Can you work these out from the model? Positions are in its coordinate system, mm. Face numbers are marked on the shaded views. A direction names the side the tool comes from. Coordinates: 2 decimals unless noted, no trailing zeros. Loops run counter-clockwise (first coordinate to the right, second up) from the corner with the lowest first, then second, coordinate; pieces in that order, holes last.
Autodesk Inventor part; units mm, degrees
ref_plane "XZ Plane" through (0, 0, 0) normal (0, 1, 0) x (-1, 0, 0)
ref_plane "XY Plane" through (0, 0, 0) normal (0, 0, 1) x (1, 0, 0)
ref_plane "Work Plane1" through (30.48, 0, 0) normal (1, 0, 0) x (0, 1, 0)
sketch "Sketch1" plane through (30.48, 0, 0) normal (1, 0, 0) x (0, 1, 0)
  line L0 (-20.1241, -2.3129) -> (-38.2674, 53.7867)
  line L1 (-38.2674, 53.7867) -> (-31.5623, 117.8336)
  line L2 (-31.5623, 117.8336) -> (-5.4691, 117.8336)
  line L3 (-5.4691, 117.8336) -> (117.3937, -58.5065)
  line L4 (117.3937, -58.5065) -> (101.0815, -66.2557)
  line L5 (19.6952, -2.3129) -> (-20.1241, -2.3129)
  line L6 (101.0815, -66.2557) -> (43.3079, -39.3441)
  line L7 (43.3079, -39.3441) -> (19.6952, -2.3129)
  line L8 (-37.8354, 57.9131) -> (-33.5614, 98.738)
  point P0 (0, 0)
  point P1 (-12.6907, 108.8336)
  point P2 (0, 0)
  dimension "d1" = 9
  dimension "d2" = 39.8192
  dimension "d3" = 107.922
  dimension "d5" = 56.0996
  dimension "d6" = 84.023
  dimension "d7" = 64.0469
  dimension "d8" = 26.0932
  dimension "d9" = 55.134
  dimension "d10" = 176.3401
  dimension "d11" = 37.0312
  dimension "d12" = 26.9116
  dimension "d13" = 18.8716
  dimension "d14" = 111.1466
extrude "Extrusion1" add sketch "Sketch1" along normal blind 3.175
ref_plane "Work Plane2" through (-30.48, 0, 0) normal (1, 0, 0) x (0, 1, 0)
sketch "Sketch2" plane through (-30.48, 0, 0) normal (1, 0, 0) x (0, 1, 0)
  line L0 (-20.1241, -2.3129) -> (19.6952, -2.3129)
  line L1 (19.6952, -2.3129) -> (43.3079, -39.3441)
  line L2 (43.3079, -39.3441) -> (101.0815, -66.2557)
  line L3 (101.0815, -66.2557) -> (117.3937, -58.5065)
  line L4 (117.3937, -58.5065) -> (-5.4691, 117.8336)
  line L5 (-5.4691, 117.8336) -> (-31.5623, 117.8336)
  line L6 (-31.5623, 117.8336) -> (-38.2674, 53.7867)
  line L7 (-38.2674, 53.7867) -> (-20.1241, -2.3129)
  point P0 (0, 0)
extrude "Extrusion2" add sketch "Sketch2" against normal blind 3.175
sketch "Sketch3" plane through (0, 0, 0) normal (0, 0, 1) x (1, 0, 0)
  line L0 (-30.48, -12.7) -> (30.48, -12.7)
  line L1 (30.48, -12.7) -> (30.48, 32.385)
  line L2 (30.48, 32.385) -> (-30.48, 32.385)
  line L3 (-30.48, 32.385) -> (-30.48, -12.7)
  line L4 (-30.48, 117.3937) -> (-30.48, -5.4691)
  line L5 (30.48, 117.3937) -> (30.48, -5.4691)
  point P0 (0, 0)
  dimension "d20" = 12.7
  dimension "d21" = 32.385
extrude "Extrusion3" add sketch "Sketch3" along normal blind 3.175
properties part number "ShoulderBoundingBox"
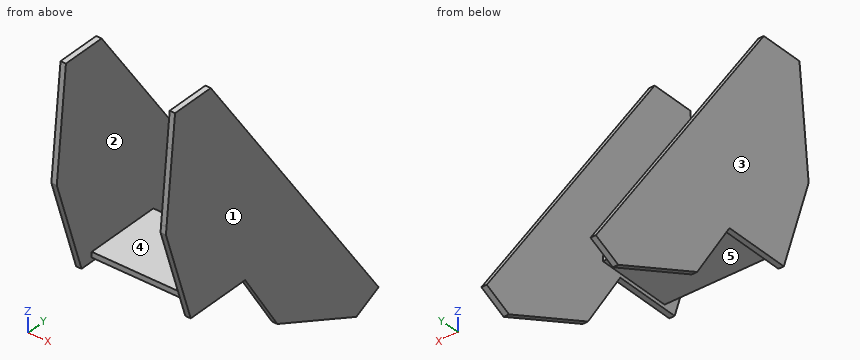
Item 1: I'm going to push flat-ended pins straight in: P1, Ø1, axis at x = -32, y = 7.5, coming from the -Z side; P2, Ø8, axis at x = 17.5, y = 4.5, coming from the +Z side (3 decimals); P3, Ø3.5, axis at x = 9, z = 1, coming from the +Y side (3 decimals). Where does each tip first touch, or does it pass through?
Results are:
P1: stops at z = -2.31
P2: stops at z = 3.175
P3: stops at y = 32.385
Item 2: We'd pull the mould along X, two halves only. Please class the marked faces 1, 2 and 3: +X half, -X half, draft (parallel to the pull), parting line (faces both ways), or undercut.
Results are:
face 1: +X half
face 2: undercut
face 3: -X half
Item 3: On a 3-axis mill with a long thin cutter (end or side, diameter ignored), from which of +Z, -Z, +X, -X, +Y, -Y can I reach the whole of each face in a straight line? I mean the marked faces 4 and 5. Say none if no direction works.
Results are:
face 4: +Z, +Y, -Y
face 5: -Z, +Y, -Y
Item 4: Suppose I cut it at A-A, the plane y = -15.5. Please give me the cut outline in (x, z) (3 decimals).
Results are:
outline: (-33.655, -2.313) - (-30.48, -2.313) - (-30.48, 117.834) - (-33.655, 117.834) - close; (30.48, -2.313) - (33.655, -2.313) - (33.655, 117.834) - (30.48, 117.834) - close
Item 5: Suppose I cut it at D-D, the plane x = -14. Please give me the cut outline in (y, z) (3 decimals).
Results are:
outline: (-12.7, 0) - (32.385, 0) - (32.385, 3.175) - (-12.7, 3.175) - close
Item 6: Suppose I cut it at B-B, the plane z = -37. Please give me the cut outline in (x, y) (3 decimals), plus the area to 3 significant figures.
Results are:
outline: (-33.655, 41.813) - (-30.48, 41.813) - (-30.48, 102.409) - (-33.655, 102.409) - close; (30.48, 41.813) - (33.655, 41.813) - (33.655, 102.409) - (30.48, 102.409) - close
area: 385 mm2
Item 7: I need wall thicknesses on line 1 along X through (y, z) = (56, -16) (3 decimals); line 2 along Z through (x, y) = (6, 17.5) (3 decimals). Which ranges of each line are inside material? Lowest first, please.
Results are:
line 1: x = -33.655 to -30.48, 30.48 to 33.655
line 2: z = 0 to 3.175
Item 8: Suppose I cut it at C-C, the plane y = 9. Please give me the cut outline in (x, z) (3 decimals).
Results are:
outline: (-33.655, -2.313) - (-30.48, -2.313) - (-30.48, 0) - (30.48, 0) - (30.48, -2.313) - (33.655, -2.313) - (33.655, 97.067) - (30.48, 97.067) - (30.48, 3.175) - (-30.48, 3.175) - (-30.48, 97.067) - (-33.655, 97.067) - close
